```python
from build123d import *

# Parameters (mm, degrees)
SKETCH1_W           = 50.8
SKETCH1_H           = 65.000000038
SKETCH1_R           = 2.5
EXTRUDE_5_DEPTH     = 7.5
SKETCH1_3_W         = 50.8
SKETCH1_3_H         = 10
BOSS_EXTRUDE1_DEPTH = 13.63
BOSS_EXTRUDE2_START = 13.63
SKETCH1_4_R         = 2.5
SKETCH1_4_R_2       = 32
SKETCH1_4_W         = 50.8
SKETCH1_4_H         = 10
BOSS_EXTRUDE2_DEPTH = 10
CHAMFER1_SIZE       = 10
CHAMFER1_SIZE_2     = 27.474774195
FILLET1_R           = 5


with BuildPart() as part:
    # Sketch1 → 5 (new body)
    with BuildSketch(Plane.XY):
        with Locations((0, 87.638385637)):
            Rectangle(SKETCH1_W, SKETCH1_H)
        with Locations((-11.25, 70.138385656)):
            Circle(SKETCH1_R, mode=Mode.SUBTRACT)
        with Locations((-11.25, 105.138385656)):
            Circle(SKETCH1_R, mode=Mode.SUBTRACT)
        with Locations((11.25, 70.138385656)):
            Circle(SKETCH1_R, mode=Mode.SUBTRACT)
        with Locations((11.25, 105.138385656)):
            Circle(SKETCH1_R, mode=Mode.SUBTRACT)
    extrude(amount=EXTRUDE_5_DEPTH)

    # Sketch1<3> → Boss-Extrude1 (add)
    with BuildSketch(Plane.XY):
        with Locations((0, 50.138385618)):
            Rectangle(SKETCH1_3_W, SKETCH1_3_H)
    extrude(amount=BOSS_EXTRUDE1_DEPTH)

    # Sketch1<4> → Boss-Extrude2 (add)
    # profile 1 of 2: a face of its own
    with BuildSketch(Plane.XY.offset(BOSS_EXTRUDE2_START)):
        with BuildLine():
            Line((-25.4, 45.138385618), (-25.4, 40.138385618))
            ThreePointArc((-25.4, 40.138385618), (0, -47.5), (25.4, 40.138385618))
            Line((25.4, 40.138385618), (25.4, 45.138385618))
            Line((25.4, 45.138385618), (-25.4, 45.138385618))
        make_face()
        with Locations((-32.285427053, -18.64)):
            Circle(SKETCH1_4_R, mode=Mode.SUBTRACT)
        with Locations((-32.285427053, 18.64)):
            Circle(SKETCH1_4_R, mode=Mode.SUBTRACT)
        with Locations((0, -37.28)):
            Circle(SKETCH1_4_R, mode=Mode.SUBTRACT)
        with Locations((32.285427053, -18.64)):
            Circle(SKETCH1_4_R, mode=Mode.SUBTRACT)
        Circle(SKETCH1_4_R_2, mode=Mode.SUBTRACT)
        with Locations((32.285427053, 18.64)):
            Circle(SKETCH1_4_R, mode=Mode.SUBTRACT)
        with Locations((0, 37.28)):
            Circle(SKETCH1_4_R, mode=Mode.SUBTRACT)
    # profile 2 of 2: a face of its own
    with BuildSketch(Plane.XY.offset(BOSS_EXTRUDE2_START)):
        with Locations((0, 50.138385618)):
            Rectangle(SKETCH1_4_W, SKETCH1_4_H)
    extrude(amount=BOSS_EXTRUDE2_DEPTH)

    # Chamfer1
    # the kernel refuses this chamfer: 27.474774195, 10 mm, written as the material it adds along each edge
    with BuildSketch(Plane(origin=(-25.4, 55.138385618, 7.5), x_dir=(0, 0.9950833631817486, -0.0990409022520505), z_dir=(1, 0, 0))) as chamfer1_piece_1_section:
        Polygon((CHAMFER1_SIZE * 0.995083363182, CHAMFER1_SIZE * 0.0990409022521), (-CHAMFER1_SIZE_2 * 0.0990409022504, CHAMFER1_SIZE_2 * 0.995083363165), (0, 0), align=None)
    chamfer1_piece_1 = extrude(amount=50.8, mode=Mode.PRIVATE)
    chamfer1_piece_1 = split(chamfer1_piece_1, bisect_by=Plane(origin=(0, 58.754193251, 23.63), z_dir=(0, 0, -1)), keep=Keep.TOP, mode=Mode.PRIVATE)
    add(chamfer1_piece_1)

    # Fillet1
    fillet1_edges = [part.edges().sort_by_distance(p)[0] for p in [
        (0, 59.267545739, 23.63),
    ]]
    fillet(fillet1_edges, radius=FILLET1_R)


solid = part.part
```
The model under review builds one solid part; all positions refer to its coordinate system, in mm. A direction names the side the tool comes from. Round coordinates to 2 decimals unless told otherwise and drop trailing zeros. Loops run counter-clockwise (first coordinate to the right, second up) from the corner with the lowest first, then second, coordinate; pieces in that order, holes last. Notation, with made-up numbers: (-36.75, 61) - (-19.75, 61) arc R17 cw to (-19.75, 93) - close; hole circle Ø9 at (38.25, 57). An arc over 180 degrees is marked (long way). Use a Markdown table: item, result. Add a question column.
Q1. For probe 1 along Y at (x, z) = (11.25, 4.25); probe 2 along Z at (x, y) = (38, 19.5); probe 3 along Y at (x, z) = (16.5, 14.25), list the stretches that pass through material, from the lowest coordinate up.
Q2. Add section D-D (z = 17.75). State the section outline as (x, y) points, plus the area to 3 significant figures.
Q3. Add section C-C (x = -19.5). State the section outline as (y, z) points.
Q4. Add section B-B (y = 0). State the section outline as (x, z) points, plus the area to 3 significant figures.
Q5. The part is to be moulded in two halves that separate along X. For faces 1 (the face through (-0.54, 34.84, 18.56)), 2 (the face through (22, 28, 23.63)), 3 (the face through (-1.71, -47.47, 18.56)), 4 (the face through (34.595, -19.598, 18.56)), say which applies: pulls with the +X half, pulls with the -X half, needs draft (parallel to the pull), parting line crosses it, or undercut.
Q6. Machinability: for faces 5 (the face through (1.34, -35.17, 18.56)), 6 (the face through (10, -31, 13.63)), 7 (the face through (-25.4, 70, 7)), 8 (the face through (0, 93, 7.5)), which of the approach directions +Z, -Z, +X, -X, +Y, -Y give a long, thin tool a straight path to every point of the face, cutting with its end or side? Answer none if there is none.
Q7. Insertion check: pin 1 Ø4 at (x, y) = (0, 37.28) entering from -Z; pin 2 Ø7 at (y, z) = (80, 6) entering from -X; pin 3 Ø6.5 at (x, y) = (-32.29, -18.64) entering from -Z; pin 4 Ø1.5 at (x, z) = (-16, 20) entering from +Y. Each pin has a flat end and moves straight along its axis. Give the tip position at first contact, or say it passes through.
Q8. Add section A-A (x = 0). State the section outline as (y, z) points, plus the area to 3 significant figures.
Worked answers:
| question | item | result |
|---|---|---|
| 1 | probe 1 | 45.14 to 67.64, 72.64 to 102.64, 107.64 to 120.14 |
| 1 | probe 2 | 13.63 to 23.63 |
| 1 | probe 3 | -44.54 to -27.42, 27.42 to 62.68 |
| 2 | outline | (-25.4, 40.14) arc R47.5 ccw (long way) to (25.4, 40.14) - (25.4, 61.41) - (-25.4, 61.41) - close; hole circle Ø5 at (-32.29, -18.64); hole circle Ø5 at (-32.29, 18.64); hole circle Ø64 at (0, 0); hole circle Ø5 at (0, -37.28); hole circle Ø5 at (0, 37.28); hole circle Ø5 at (32.29, -18.64); hole circle Ø5 at (32.29, 18.64) |
| 2 | area | 4,580 mm² |
| 3 | outline | (-43.31, 13.63) - (-25.37, 13.63) - (-25.37, 23.63) - (-43.31, 23.63) - close; (25.37, 13.63) - (45.14, 13.63) - (45.14, 0) - (120.14, 0) - (120.14, 7.5) - (65.14, 7.5) - (60.46, 20.34) arc R5 ccw to (55.77, 23.63) - (25.37, 23.63) - close |
| 4 | outline | (-47.5, 13.63) - (-32, 13.63) - (-32, 23.63) - (-47.5, 23.63) - close; (32, 13.63) - (47.5, 13.63) - (47.5, 23.63) - (32, 23.63) - close |
| 4 | area | 310 mm² |
| 5 | face 1 | undercut |
| 5 | face 2 | needs draft |
| 5 | face 3 | parting line crosses it |
| 5 | face 4 | undercut |
| 6 | face 5 | +Z, -Z |
| 6 | face 6 | -Z, +X, -X, -Y |
| 6 | face 7 | +Z, -Z, -X, +Y |
| 6 | face 8 | +Z, +X, -X, +Y |
| 7 | pin 1 | through |
| 7 | pin 2 | x = -25.4 |
| 7 | pin 3 | z = 13.63 |
| 7 | pin 4 | y = 60.86 |
| 8 | outline | (-47.5, 13.63) - (-39.78, 13.63) - (-39.78, 23.63) - (-47.5, 23.63) - close; (-34.78, 13.63) - (-32, 13.63) - (-32, 23.63) - (-34.78, 23.63) - close; (32, 13.63) - (34.78, 13.63) - (34.78, 23.63) - (32, 23.63) - close; (39.78, 13.63) - (45.14, 13.63) - (45.14, 0) - (120.14, 0) - (120.14, 7.5) - (65.14, 7.5) - (60.46, 20.34) arc R5 ccw to (55.77, 23.63) - (39.78, 23.63) - close |
| 8 | area | 1,020 mm² |
